The listing builds one solid part. Answer for the finished solid, in the listing's coordinates (mm). A direction names the side the tool comes from. Coordinates: 2 decimals unless noted, no trailing zeros. Write each loop counter-clockwise with the first axis right and the second up, starting at its lowest first coordinate (ties: lowest second). Pieces come first, ordered by that corner, then holes. Notation, with made-up numbers: M 26.25,-38.75 L 71.25,-38.75 A24 cw 71.25,-18.75 Z; hole C 16.5,62 d11. An arc over 180 degrees is marked long. Write item = value, one per line. Start each with the question number.
Autodesk Inventor part; units mm, degrees
ref_plane "YZ Plane" through (0, 0, 0) normal (1, 0, 0) x (0, 1, 0)
ref_plane "XZ Plane" through (0, 0, 0) normal (0, 1, 0) x (-1, 0, 0)
ref_plane "XY Plane" through (0, 0, 0) normal (0, 0, 1) x (1, 0, 0)
sketch "Sketch1" plane through (0, 0, 0) normal (0, 0, 1) x (1, 0, 0)
  line L0 (0, 0) -> (50.8, 0)
  line L1 (50.8, 0) -> (50.8, 69.85)
  line L2 (50.8, 69.85) -> (0, 69.85)
  line L3 (0, 69.85) -> (0, 0)
  dimension "d0" = 50.8
  dimension "d1" = 69.85
extrude "Extrusion1" add sketch "Sketch1" along normal blind 2.54
sketch "Sketch2" plane through (50.8, 0, 0) normal (1, 0, 0) x (0, 0, -1)
  line L0 (0, 0) -> (0, 69.85) construction
  line L1 (0, 69.85) -> (0, 139.7) construction
  line L2 (-2.54, 0) -> (-2.54, 69.85) construction
  line L3 (-2.54, 69.85) -> (-42.8679, 139.7)
  line L4 (-2.54, 69.85) -> (78.1158, 69.85) construction
  line L5 (-42.8679, 139.7) -> (-40.6682, 140.97)
  line L6 (-40.6682, 140.97) -> (0, 70.5306)
  line L7 (0, 69.85) -> (-2.54, 69.85)
  line L8 (0, 70.5306) -> (0, 69.85)
  dimension "d4" = 69.85
  dimension "d5" = 120
  dimension "d6" = 2.54
extrude "Extrusion2" add sketch "Sketch2" along normal blind 38.1 and the other way blind 88.9
fillet "Fillet1" radius 12.7 2 edges at (0, 69.85, 1.27) (50.8, 69.85, 1.27)
fillet "Fillet2" radius 3.175 4 edges at (88.9, 140.335, 41.7681) (-38.1, 140.335, 41.7681) (-38.1, 69.85, 1.27) (88.9, 69.85, 1.27)
sketch "Sketch3" plane through (0, 0, 2.54) normal (0, 0, 1) x (1, 0, 0)
  line L0 (0, 0) -> (50.8, 0)
  line L1 (0, 57.15) -> (0, 0)
  line L2 (50.8, 0) -> (50.8, 57.15)
  point P0 (12.7, 12.7)
  point P1 (38.1, 12.7)
  dimension "d13" = 12.7
  dimension "d14" = 12.7
  dimension "d15" = 12.7
  dimension "d16" = 12.7
hole "Hole1" at (12.7, 12.7, 2.54) at (38.1, 12.7, 2.54) direction (0, 0, -1) diameter 3.937 end through all
properties part number "DeliveryBoxBackstop"
1. For a pull along Y with two mould halves and no side action, classify faces 1 (the face through (24.511, 104.286, 22.422)), 2 (the face through (-38.1, 106, 21)), 3 (the face through (36.44, 11.64, 1.25)), 4 (the face through (14.446, 11.792, 1.252)) as pulls with the +Y half, pulls with the -Y half, needs draft (parallel to the pull), parting line crosses it, or undercut.
2. For faces 5 (the face through (25, 35, 2.54)), 6 (the face through (-37.19, 70.8, 1.73)), determine the directions among +Z, -Z, +X, -X, +Y, -Y from which every point of the face is accessible in a straight line to the end or side of a thin tool.
3. The part is cut by section C-C, the plane x = 8. Write down the section's boundary in (y, z).
4. The part is cut by section B-B, the plane x = 38.1. Write down the section's boundary in (y, z).
5. The part is cut by section D-D, the plane z = 6. Write down the section's boundary in (x, y), and give its area (3 significant figures).
6. Straight lines are drawn through the part: L1, parallel to X at y = 12.7, z = 1.8; L2, parallel to X at y = 12, z = 1; L3, parallel to Y at x = 12, z = 1. For each, find the intervals that lie inside material, in ascending order. Write a range as [from, to].
7. Each of these flat-tipped pins is pushed along its axis until it touches: pin 1 (10 mm diameter, centred on x = 30.5, y = 107.5, fed in from -Z); pin 2 (10 mm diameter, centred on x = 6.5, y = 28.5, fed in from +Z); pin 3 (3 mm diameter, centred on x = 48.5, z = 20.5, fed in from +Y). Where does it stop, or does it pass through?
8. The part is cut by section A-A, the plane y = 12.7. Write down the section's boundary in (x, z).
Solution:
q1.face_1 = pulls with the -Y half
q1.face_2 = needs draft
q1.face_3 = undercut
q1.face_4 = undercut
q2.face_5 = +Z, +X, -X, -Y
q2.face_6 = +Z, -Z, -X, -Y
q3.outline = M 0,0 L 70.53,0 L 140.97,40.67 L 139.7,42.87 L 69.85,2.54 L 0,2.54 Z
q4.outline = M 0,0 L 10.73,0 L 10.73,2.54 L 0,2.54 Z; M 14.67,0 L 70.53,0 L 140.97,40.67 L 139.7,42.87 L 69.85,2.54 L 14.67,2.54 Z
q5.outline = M -38.1,75.84 L 88.9,75.84 L 88.9,80.92 L -38.1,80.92 Z
q5.area = 645 mm^2
q6.L1 = [0, 10.73], [14.67, 36.13], [40.07, 50.8]
q6.L2 = [0, 10.86], [14.54, 36.26], [39.94, 50.8]
q6.L3 = [0, 10.86], [14.54, 72.26]
q7.pin_1 = 18.46
q7.pin_2 = 2.54
q7.pin_3 = 108.64
q8.outline = M 0,0 L 10.73,0 L 10.73,2.54 L 0,2.54 Z; M 14.67,0 L 36.13,0 L 36.13,2.54 L 14.67,2.54 Z; M 40.07,0 L 50.8,0 L 50.8,2.54 L 40.07,2.54 Z
